Verification items for this drawing (mm, ordinates from the low corner). Give positions to 0.01 mm unless a question says otherwise; leave off trailing zeros. Order: outer loops, then holes, each group sorted by start corner. A loop starts at its lowest first (then second) coordinate and runs counter-clockwise, first axis right, second up. Notation, with made-up numbers: (66, -16.75) -> (77, -16.75) arc R8 cw to (77, -12.75) -> close; hole circle Ø7 at (-6, -11). An arc over 180 degrees is marked (long way). One line per question, with ' | ' between items.
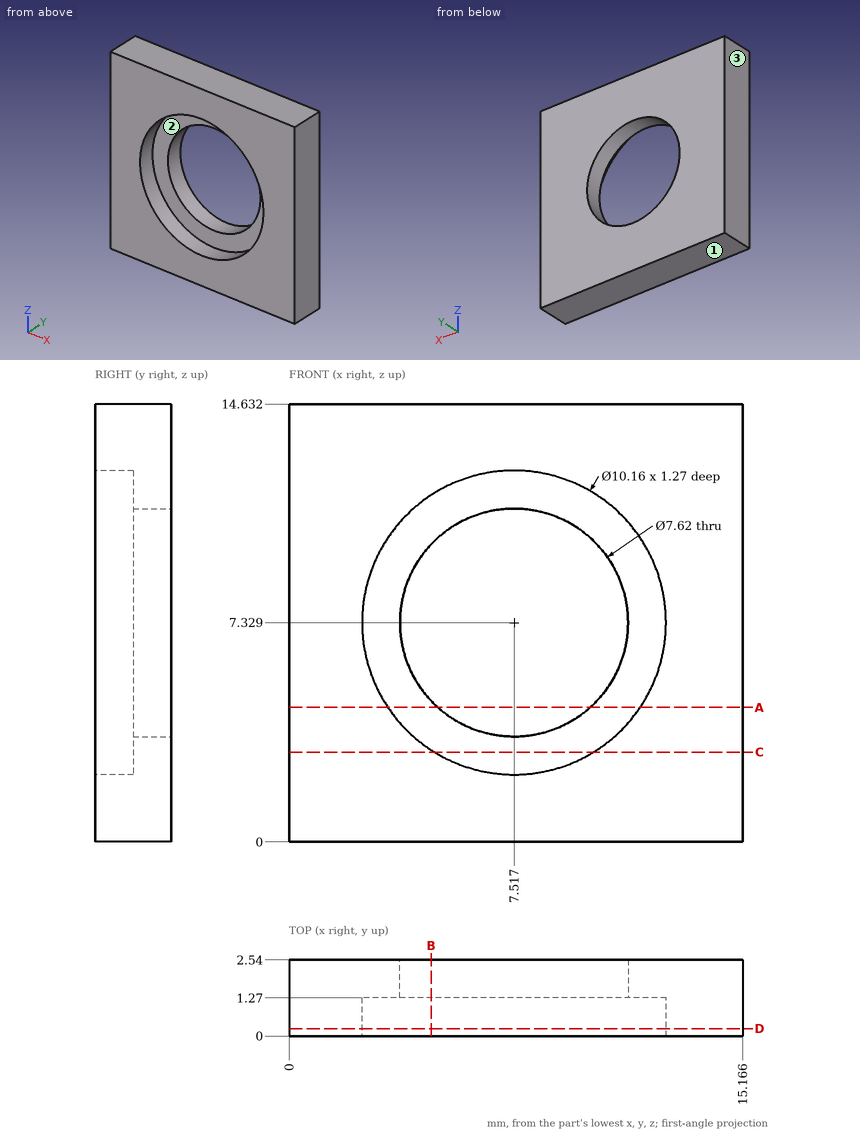
Q1. Section check D-D (y = 0.25). Enter the section's corners in (x, z) (1 decimal).
Result sheet:
outline: (0, 0) -> (15.2, 0) -> (15.2, 14.6) -> (0, 14.6) -> close; hole circle Ø10.2 at (7.5, 7.3)
Q2. Section check B-B (x = 4.75). Enter the section's corners in (y, z), and give its area (3 significant figures).
Result sheet:
outline: (0, 0) -> (2.54, 0) -> (2.54, 4.71) -> (1.27, 4.71) -> (1.27, 3.07) -> (0, 3.07) -> close; (0, 11.59) -> (1.27, 11.59) -> (1.27, 9.95) -> (2.54, 9.95) -> (2.54, 14.63) -> (0, 14.63) -> close | area: 19.7 mm2
Q3. Depth check by flat-ended pin: pin 1 Ø2 at (x, z) = (9.5, 8) entering from +Y. Enter the tip coordinate at first touch or a pass-through.
Result sheet:
pin 1: passes through
Q4. Thickness scan on line 1 (Y direction, x = 3, z = 7.75); line 2 (X direction, y = 1.75, z = 4.75) (1 decimal); line 3 (Z direction, x = 3.5, y = 1.2) (1 decimal). Record the ranges inside material, lowest first.
Result sheet:
line 1: y = 1.27 to 2.54 | line 2: x = 0 to 4.7, 10.3 to 15.2 | line 3: z = 0 to 4.2, 10.4 to 14.6
Q5. Mould release check, pull along X, two halves, no side actions. Record for the marked faces 1, 2 and 3: pulls with the +X half, pulls with the -X half, needs draft (parallel to the pull), parting line crosses it, or undercut.
Result sheet:
face 1: needs draft | face 2: undercut | face 3: pulls with the -X half
Q6. Section check A-A (z = 4.5). Enter the section's corners in (x, y) (1 decimal).
Result sheet:
outline: (0, 0) -> (3.3, 0) -> (3.3, 1.3) -> (5, 1.3) -> (5, 2.5) -> (0, 2.5) -> close; (10.1, 1.3) -> (11.7, 1.3) -> (11.7, 0) -> (15.2, 0) -> (15.2, 2.5) -> (10.1, 2.5) -> close
Q7. Section check C-C (z = 3). Enter the section's corners in (x, y) (1 decimal).
Result sheet:
outline: (0, 0) -> (4.9, 0) -> (4.9, 1.3) -> (10.2, 1.3) -> (10.2, 0) -> (15.2, 0) -> (15.2, 2.5) -> (0, 2.5) -> close
